Input: part model. Units: mm. Frame: model coordinates. A direction names the side the tool comes from. Coordinates: 2 decimals unless noted, no trailing zeros. Write each loop counter-clockwise with the first axis right and the second up, starting at its lowest first coordinate (ties: lowest second). Pieces come first, ordered by that corner, then holes. Notation, with made-up numbers: (-32.75, 77) - (7.25, 77) arc R10 cw to (7.25, 91) - close; hole circle Ø7 at (-33, 44.25). An arc over 180 degrees is marked (long way). Put each result on its own line as item: value. Start each with the question number.
1. Pin query (flat end, axial travel): pin 1 (18.5 mm diameter, centred on y = -1, z = 25, fed in from +X); pin 2 (6 mm diameter, centred on y = 0.5, z = 20.5, fed in from -X); pin 3 (6 mm diameter, centred on y = 17, z = 24, fed in from -X). Return the tip coordinate at first contact, or that it passes through.
2. Cut plane C-C, the plane x = -46.5. Return loops of the section in (y, z).
3. Pull-direction query (Y, two-part tool) for faces 4 (the flat face through (-1, 7, 46)), 5 (the cylindrical face through (-37.69, -0.96, 44.52)); classes: released by +Y, released by -Y, zero draft, split by the parting line, or undercut.
4. Access query for faces 1 (the flat face through (-40, -3.9, 40)), 2 (the flat face through (-80, -8.5, 20)), 3 (the cylindrical face through (77.5, 0.1, 44.5)). Directions: +Z, -Z, +X, -X, +Y, -Y. A direction counts if a zero-diameter tool reaches every point of the face in a straight line with its end or side. Return the directions, or none.
5. Cut plane A-A, the plane x = 40. Return loops of the section in (y, z), and give its area (3 significant figures).
6. Cut plane B-B, the plane y = 16.5. Return loops of the section in (x, z), and give its area (3 significant figures).
7. Line query: line 1 (Y direction, x = -84.5, z = 21.5); line 2 (X direction, y = 8, z = 17); line 3 (Y direction, x = -36, z = 25). Output: solid intervals per line, ascending.
from build123d import *

# Parameters (mm, degrees)
SKETCH_W        = 180
SKETCH_H        = 50
PAD_DEPTH       = 40
SKETCH001_W     = 188
SKETCH001_H     = 57
PAD001_DEPTH    = 6
SKETCH003_W     = 50
SKETCH003_H     = 17
POCKET_DEPTH    = 38
SKETCH004_R     = 2.5
POCKET001_DEPTH = 46.001
FILLET_R        = 5
FILLET001_R     = 2
POCKET002_DEPTH = 5
SKETCH006_R     = 6
POCKET003_DEPTH = 8.001


with BuildPart() as part:
    # Sketch → Pad (new body)
    with BuildSketch(Plane.XY):
        Rectangle(SKETCH_W, SKETCH_H)
    extrude(amount=PAD_DEPTH)

    # Sketch001 (on Face6 of Pad) → Pad001 (join)
    with BuildSketch(Plane.XY.offset(40)):
        Rectangle(SKETCH001_W, SKETCH001_H)
    extrude(amount=PAD001_DEPTH)

    # Sketch003 (on Face11 of Pad001) → Pocket (cut)
    with BuildSketch(Plane(origin=(0, 0, 0), x_dir=(1, 0, 0), z_dir=(0, 0, -1))):
        Polygon((-85, -20), (85, -20), (85, -13.5), (66, -13.5), (66, 13.5), (85, 13.5), (85, 20), (-85, 20), (-85, 13.5), (-66, 13.5), (-66, -13.5), (-85, -13.5), align=None)
        with Locations((-96, 0)):
            Rectangle(SKETCH003_W, SKETCH003_H)
        with Locations((96, 0)):
            Rectangle(SKETCH003_W, SKETCH003_H)
    extrude(amount=-POCKET_DEPTH, mode=Mode.SUBTRACT)

    # Sketch004 (on Face5 of Pocket) → Pocket001 (cut, through all)
    with BuildSketch(Plane.XY.offset(46)):
        with Locations((-80, 0)):
            Circle(SKETCH004_R)
        with Locations((-60, 0)):
            Circle(SKETCH004_R)
        with Locations((-40, 0)):
            Circle(SKETCH004_R)
        with Locations((-20, 0)):
            Circle(SKETCH004_R)
        Circle(SKETCH004_R)
        with Locations((20, 0)):
            Circle(SKETCH004_R)
        with Locations((40, 0)):
            Circle(SKETCH004_R)
        with Locations((60, 0)):
            Circle(SKETCH004_R)
        with Locations((80, 0)):
            Circle(SKETCH004_R)
    extrude(amount=-POCKET001_DEPTH, mode=Mode.SUBTRACT)

    # Fillet
    fillet_edges = [part.edges().sort_by_distance(p)[0] for p in [
        (94, 28.5, 43),
        (94, -28.5, 43),
        (-94, -28.5, 43),
        (-94, 28.5, 43),
    ]]
    fillet(fillet_edges, radius=FILLET_R)

    # Fillet001
    fillet001_edges = [part.edges().sort_by_distance(p)[0] for p in [
        (-90, 16.75, 0),
        (-80.5, 8.5, 0),
        (-71, 0, 0),
        (-80.5, -8.5, 0),
        (-90, -16.75, 0),
        (0, -25, 0),
        (90, -16.75, 0),
        (80.5, -8.5, 0),
        (71, 0, 0),
        (80.5, 8.5, 0),
        (90, 16.75, 0),
        (0, 25, 0),
        (-75.5, -13.5, 0),
        (-66, 0, 0),
        (-75.5, 13.5, 0),
        (-85, 16.75, 0),
        (0, 20, 0),
        (85, 16.75, 0),
        (75.5, 13.5, 0),
        (66, 0, 0),
        (75.5, -13.5, 0),
        (85, -16.75, 0),
        (0, -20, 0),
        (-85, -16.75, 0),
        (-90, -8.5, 19),
        (-90, 25, 20),
        (-90, 8.5, 19),
        (90, -25, 20),
        (-90, -25, 20),
        (90, 25, 20),
        (90, -8.5, 19),
        (90, 8.5, 19),
        (-66, 13.5, 19),
        (-66, -13.5, 19),
        (66, -13.5, 19),
        (66, 13.5, 19),
    ]]
    fillet(fillet001_edges, radius=FILLET001_R)

    # Sketch005 (on Face73 of Fillet001) → Pocket002 (cut)
    with BuildSketch(Plane(origin=(0, 0, 38), x_dir=(1, 0, 0), z_dir=(0, 0, -1))):
        Polygon((-77.748334, -3.9), (-75.496668, 0), (-77.748334, 3.9), (-82.251666, 3.9), (-84.503332, 0), (-82.251666, -3.9), align=None)
        Polygon((-57.748334, -3.9), (-55.496668, 0), (-57.748334, 3.9), (-62.251666, 3.9), (-64.503332, 0), (-62.251666, -3.9), align=None)
        Polygon((-37.748334, -3.9), (-35.496668, 0), (-37.748334, 3.9), (-42.251666, 3.9), (-44.503332, 0), (-42.251666, -3.9), align=None)
        Polygon((-17.748334, -3.9), (-15.496668, 0), (-17.748334, 3.9), (-22.251666, 3.9), (-24.503332, 0), (-22.251666, -3.9), align=None)
        Polygon((2.251666, -3.9), (4.503332, 0), (2.251666, 3.9), (-2.251666, 3.9), (-4.503332, 0), (-2.251666, -3.9), align=None)
        Polygon((22.251666, -3.9), (24.503332, 0), (22.251666, 3.9), (17.748334, 3.9), (15.496668, 0), (17.748334, -3.9), align=None)
        Polygon((42.251666, -3.9), (44.503332, 0), (42.251666, 3.9), (37.748334, 3.9), (35.496668, 0), (37.748334, -3.9), align=None)
        Polygon((62.251666, -3.9), (64.503332, 0), (62.251666, 3.9), (57.748334, 3.9), (55.496668, 0), (57.748334, -3.9), align=None)
        Polygon((82.251666, -3.9), (84.503332, 0), (82.251666, 3.9), (77.748334, 3.9), (75.496668, 0), (77.748334, -3.9), align=None)
    extrude(amount=-POCKET002_DEPTH, mode=Mode.SUBTRACT)

    # Sketch006 (on Face152 of Pocket002) → Pocket003 (cut, through all)
    with BuildSketch(Plane(origin=(0, 0, 38), x_dir=(1, 0, 0), z_dir=(0, 0, -1))):
        with Locations((-10, -13)):
            Circle(SKETCH006_R)
    extrude(amount=-POCKET003_DEPTH, mode=Mode.SUBTRACT)


solid = part.part
Report:
1. pin 1: stops at x = 89.98
1. pin 2: stops at x = -71
1. pin 3: stops at x = -90
2. outline: (-28.5, 40) - (-25, 40) - (-25, 2) arc R2 ccw to (-23, 0) - (-22, 0) arc R2 ccw to (-20, 2) - (-20, 38) - (20, 38) - (20, 2) arc R2 ccw to (22, 0) - (23, 0) arc R2 ccw to (25, 2) - (25, 40) - (28.5, 40) - (28.5, 46) - (-28.5, 46) - close
3. face 4: zero draft
3. face 5: undercut
4. face 1: -Z
4. face 2: -Z, -X
4. face 3: +Z, -Z
5. outline: (-28.5, 40) - (-25, 40) - (-25, 2) arc R2 ccw to (-23, 0) - (-22, 0) arc R2 ccw to (-20, 2) - (-20, 38) - (-3.9, 38) - (-3.9, 43) - (-2.5, 43) - (-2.5, 46) - (-28.5, 46) - close; (2.5, 43) - (3.9, 43) - (3.9, 38) - (20, 38) - (20, 2) arc R2 ccw to (22, 0) - (23, 0) arc R2 ccw to (25, 2) - (25, 40) - (28.5, 40) - (28.5, 46) - (2.5, 46) - close
5. area: 765 mm^2
6. outline: (-94, 40) - (-90, 40) - (-90, 2) arc R2 ccw to (-88, 0) - (-87, 0) arc R2 ccw to (-85, 2) - (-85, 38) - (-14.87, 38) - (-14.87, 46) - (-94, 46) - close; (-5.13, 38) - (85, 38) - (85, 2) arc R2 ccw to (87, 0) - (88, 0) arc R2 ccw to (90, 2) - (90, 40) - (94, 40) - (94, 46) - (-5.13, 46) - close
6. area: 1,790 mm^2
7. line 1: y = -25 to -20, -13.5 to -8.5, 8.5 to 13.5, 20 to 25
7. line 2: x = -71 to -66, 66 to 71
7. line 3: y = -25 to -20, 20 to 25
